Build history of the part. All positions in model axes, mm. Face numbers are marked on the shaded views. A direction names the side the tool comes from. Coordinates: 2 decimals unless noted, no trailing zeros. Order: outer loops, then holes, each group sorted by start corner. A loop starts at its lowest first (then second) coordinate and runs counter-clockwise, first axis right, second up. Notation, with made-up numbers: (13, 89) - (66, 89) arc R11 ccw to (66, 97) - close; hole circle Ø4 at (51.25, 27). An arc over 180 degrees is marked (long way). Write each question's results on one line, items separated by ' | '.
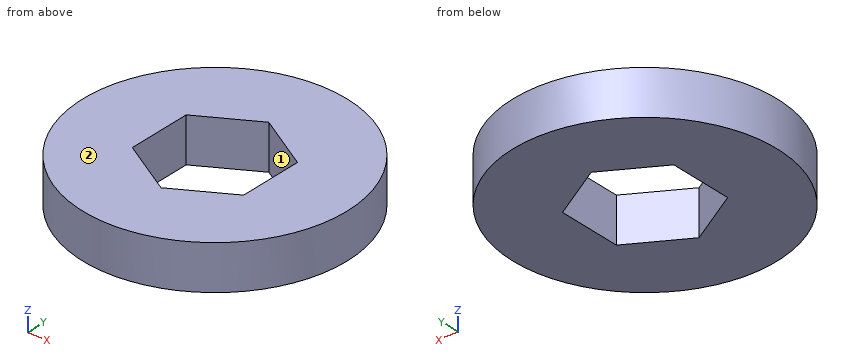
from build123d import *

# Parameters (mm, degrees)
SKETCH1_R           = 11.85
BOSS_EXTRUDE1_DEPTH = 4
CUT_EXTRUDE1_DEPTH  = 18.229190347
SCALE1_SCALE        = 0.4


with BuildPart() as part:
    # Sketch1 → Boss-Extrude1 (new body)
    with BuildSketch(Plane.XY):
        Circle(SKETCH1_R)
    extrude(amount=BOSS_EXTRUDE1_DEPTH)

    # Sketch2 → Cut-Extrude1 (cut, through all)
    with BuildSketch(Plane(origin=(0, 0, 0), x_dir=(-1, 0, 0), z_dir=(0, 0, -1))):
        Polygon((0, 5.773502692), (-5, 2.886751346), (-5, -2.886751346), (0, -5.773502692), (5, -2.886751346), (5, 2.886751346), align=None)
    extrude(amount=-CUT_EXTRUDE1_DEPTH, mode=Mode.SUBTRACT)


with BuildPart() as part_1:
    # Scale1: scaled about (0, 0, 2)
    add(part.part.scale(SCALE1_SCALE).moved(Location((0, 0, 1.2))))


solid = part_1.part
1. Band-saw the part on A-A on y = 0. Give the cut face in (x, z), then the cut area to 3 significant figures.
Solved:
outline: (-4.74, 1.2) - (-2, 1.2) - (-2, 2.8) - (-4.74, 2.8) - close; (2, 1.2) - (4.74, 1.2) - (4.74, 2.8) - (2, 2.8) - close | area: 8.77 mm2
2. Band-saw the part on C-C on z = 1.9. Give the cut face in (x, y).
Solved:
outline: circle Ø9.48 at (0, 0); hole (-2, -1.15) - (0, -2.31) - (2, -1.15) - (2, 1.15) - (0, 2.31) - (-2, 1.15) - close
3. Band-saw the part on B-B on x = 1.25. Give the cut face in (y, z).
Solved:
outline: (-4.57, 1.2) - (-1.59, 1.2) - (-1.59, 2.8) - (-4.57, 2.8) - close; (1.59, 1.2) - (4.57, 1.2) - (4.57, 2.8) - (1.59, 2.8) - close
4. Tool access for the marked faces 1 and 2: list every direction of +Z, -Z, +X, -X, +Y, -Y with a clear straight run to the whole face (end or side of a thin tool).
Solved:
face 1: +Z, -Z | face 2: +Z, +X, -X, +Y, -Y
5. Probe line 1 (Y direction, x = -1.75, z = 2.2); line 2 (Y direction, x = -0.5, z = 1.9); line 3 (X direction, y = -0.75, z = 2.25). List the from-to ranges inside material, lowest first.
Solved:
line 1: y = -4.41 to -1.3, 1.3 to 4.41 | line 2: y = -4.71 to -2.02, 2.02 to 4.71 | line 3: x = -4.68 to -2, 2 to 4.68
6. Band-saw the part on D-D on y = -3.5. Give the cut face in (x, z).
Solved:
outline: (-3.2, 1.2) - (3.2, 1.2) - (3.2, 2.8) - (-3.2, 2.8) - close
